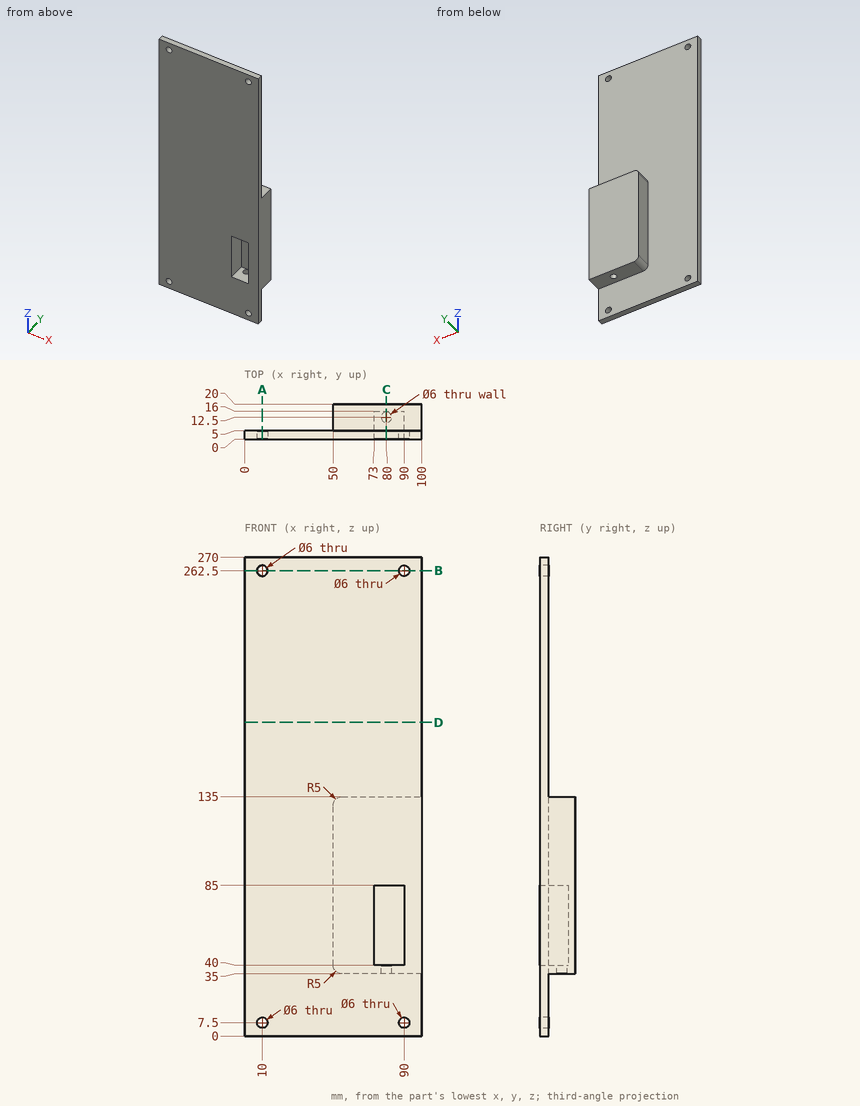
Input: dimensioned drawing with shaded views. Units: mm. Origin: part minimum x, y, z. Coordinates: 2 decimals unless noted, no trailing zeros. Order: outer loops, then holes, each group sorted by start corner. A loop starts at its lowest first (then second) coordinate and runs counter-clockwise, first axis right, second up. Notation, with made-up numbers: (42, 71.5) - (54, 71.5) arc R12 ccw to (54, 83.5) - close; hole circle Ø3 at (-17, -34). An arc over 180 degrees is marked (long way). One line per item, written item: value.
1) Contact query for flat-ended pins moving along their axis: pin 1 (5 mm diameter, centred on x = 80, y = 12.5, fed in from -Z); pin 2 (5 mm diameter, centred on y = 11, z = 54.5, fed in from -X); pin 3 (3.5 mm diameter, centred on x = 10, z = 7.5, fed in from -Y); pin 4 (4 mm diameter, centred on x = 83, y = 10, fed in from +Z). Output: stop coordinate, or through.
Computed values:
pin 1: stops at z = 85
pin 2: stops at x = 50
pin 3: passes through
pin 4: stops at z = 135
2) Cut plane B-B on z = 262.5. Output: boundary loops of the cut face in (x, y).
Computed values:
outline: (0, 0) - (7, 0) - (7, 5) - (0, 5) - close; (13, 0) - (87, 0) - (87, 5) - (13, 5) - close; (93, 0) - (100, 0) - (100, 5) - (93, 5) - close
3) Ray query, line 1 (X direction, y = 3.6, z = 262.5); line 2 (Z direction, x = 10, y = 1.9); line 3 (X direction, y = 5.5, z = 53). Return the intervals inside material, ascending. Write a range as [from, to].
Computed values:
line 1: x = [0, 7], [13, 87], [93, 100]
line 2: z = [0, 4.5], [10.5, 259.5], [265.5, 270]
line 3: x = [50, 73], [90, 100]
4) Cut plane A-A on x = 10. Output: boundary loops of the cut face in (y, z).
Computed values:
outline: (0, 0) - (5, 0) - (5, 4.5) - (0, 4.5) - close; (0, 10.5) - (5, 10.5) - (5, 259.5) - (0, 259.5) - close; (0, 265.5) - (5, 265.5) - (5, 270) - (0, 270) - close
5) Cut plane D-D on z = 177. Output: boundary loops of the cut face in (x, y), plus the area to 3 significant figures.
Computed values:
outline: (0, 0) - (100, 0) - (100, 5) - (0, 5) - close
area: 500 mm^2
6) Cut plane C-C on x = 80. Output: boundary loops of the cut face in (y, z).
Computed values:
outline: (0, 0) - (5, 0) - (5, 35) - (9.5, 35) - (9.5, 40) - (0, 40) - close; (0, 85) - (16, 85) - (16, 40) - (15.5, 40) - (15.5, 35) - (20, 35) - (20, 135) - (5, 135) - (5, 270) - (0, 270) - close
